```python
from build123d import *

# Parameters (mm, degrees)
F0_R           = 6.1
F1_DEPTH       = 10
F2_W           = 8.5
F2_H           = 45.4
F2_W_2         = 10
F3_DEPTH       = 10
F5_D           = 3.3
F5_CBORE_D     = 6.5
F5_CBORE_DEPTH = 3
F7_DEPTH       = 8.5
F7_DEPTH_BACK  = 18.5
F9_DEPTH       = 45.401


with BuildPart() as f1:
    # F0 (on Right) → F1 (new body)
    with BuildSketch(Plane.YZ):
        with BuildLine():
            Line((22.7, 0), (0, 0))
            Line((0, 0), (-22.7, 0))
            Line((-22.7, 0), (-10, -45))
            ThreePointArc((-10, -45), (0, -35), (10, -45))
            Line((10, -45), (22.7, 0))
        make_face()
        with Locations((0, -10)):
            Circle(F0_R, mode=Mode.SUBTRACT)
        with BuildLine():
            ThreePointArc((10, -45), (0, -35), (-10, -45))
            ThreePointArc((-10, -45), (0, -55), (10, -45))
        make_face()
        with Locations((0, -45)):
            Circle(F0_R, mode=Mode.SUBTRACT)
    extrude(amount=F1_DEPTH)

    # F2 (on face) → F3 (join)
    with BuildSketch(Plane.XY):
        with Locations((14.25, 0)):
            Rectangle(F2_W, F2_H)
        with Locations((5, 0)):
            Rectangle(F2_W_2, F2_H)
        with Locations((-4.25, 0)):
            Rectangle(F2_W, F2_H)
    extrude(amount=F3_DEPTH)

    # F5 (through all)
    with Locations(Plane(origin=(0, 0, 0), x_dir=(1, 0, 0), z_dir=(0, 0, -1))):
        with Locations((-5, 10), (15, 10), (15, -10), (-5, -10)):
            CounterBoreHole(F5_D / 2, F5_CBORE_D / 2, F5_CBORE_DEPTH)

    # F6 (on face) → F7 (join, two sides)
    with BuildSketch(Plane.YZ.offset(10)) as f7_sk:
        with BuildLine():
            Line((21.1, 0), (8.4, -45))
            ThreePointArc((8.4, -45), (0, -53.4), (-8.4, -45))
            Line((-8.4, -45), (-21.1, 0))
            Line((-21.1, 0), (-22.7, 0))
            Line((-22.7, 0), (-10, -45))
            ThreePointArc((-10, -45), (0, -55), (10, -45))
            Line((10, -45), (22.7, 0))
            Line((22.7, 0), (21.1, 0))
        make_face()
    extrude(amount=F7_DEPTH)
    extrude(f7_sk.sketch, amount=-F7_DEPTH_BACK)

    # F8 (on face) → F9 (cut, through all)
    with BuildSketch(Plane.XZ.offset(22.7)):
        Polygon((0, -45), (-8.5, 0), (-8.5, -58.9339546859), (18.5, -58.9339546859), (18.5, 0), (10, -45), (10, -55), (0, -55), align=None)
    extrude(amount=-F9_DEPTH, mode=Mode.SUBTRACT)


solid = f1.part
```
The listing builds one solid part. Answer for the finished solid, in the listing's coordinates (mm). A direction names the side the tool comes from. Round coordinates to 2 decimals unless told otherwise and drop trailing zeros. Write each loop counter-clockwise with the first axis right and the second up, starting at its lowest first coordinate (ties: lowest second). Pieces come first, ordered by that corner, then holes. Notation, with made-up numbers: (-29.5, 9) -> (-12.5, 9) arc R16 ccw to (-12.5, 14) -> close; hole circle Ø6 at (-22, 34.25). An arc over 180 degrees is marked (long way). Answer as a JSON object with one key per item and string values. Group by question number.
Q1. Straight lines are drawn through the part: line 1 along Y through (x, z) = (-5, 2.1); line 2 along X through (y, z) = (10, 1); line 3 along X through (y, z) = (-10, 6.75). For each, find the intervals that lie inside material, in ascending order.
Q2. Section D-D (x = 15) is taken. Write down the section's boundary in (y, z).
Q3. Each of these flat-tipped pins is pushed along its axis until it touches: pin 1 Ø4 at (y, z) = (8, -28) entering from -X; pin 2 Ø2 at (x, y) = (15, 10) entering from +Z; pin 3 Ø2.5 at (x, y) = (-4.5, 7) entering from -Z; pin 4 Ø4 at (x, y) = (-5, -10) entering from -Z. Where does it stop, or does it pass through?
Q4. Section B-B (x = 8.25) is taken. Write down the section's boundary in (y, z).
Q5. Section C-C (z = -10) is taken. Write down the section's boundary in (x, y).
Q6. Which of the six approach directions +Z, -Z, +X, -X, +Y, -Y give full straight-line access (tool end or side, diameter ignored) to faces 1 (the face through (-3.25, 16.25, -17.18)), 2 (the face through (13.476, 10.632, 6.549)), 3 (the face through (16.4, 11.4, 3)), 4 (the face through (13.25, 16.25, -17.19))?
Q7. Section A-A (y = 0) is taken. Write down the section's boundary in (x, z), plus the area to 3 significant figures.
Q8. Determine the mould class of faces 5 (the face through (-8.5, 0, 5)), 6 (the face through (12.3, -17.48, -12.82)), 7 (the face through (4.811, 17.672, -17.815)) for opening direction Y: pulls with the +Y half, pulls with the -Y half, needs draft (parallel to the pull), parting line crosses it, or undercut.
Check values:
{
 "1": {"line 1": "-22.7 to -13.25, -6.75 to 6.75, 13.25 to 22.7", "line 2": "-8.5 to -8.25, -1.75 to 11.75, 18.25 to 18.5", "line 3": "-8.5 to -6.65, -3.35 to 13.35, 16.65 to 18.5"},
 "2": {"outline": "(-22.7, 0) -> (-17.47, -18.53) -> (-15.87, -18.53) -> (-21.1, 0) -> (-13.25, 0) -> (-13.25, 3) -> (-11.65, 3) -> (-11.65, 10) -> (-22.7, 10) -> close; (-8.35, 3) -> (-6.75, 3) -> (-6.75, 0) -> (6.75, 0) -> (6.75, 3) -> (8.35, 3) -> (8.35, 10) -> (-8.35, 10) -> close; (11.65, 3) -> (13.25, 3) -> (13.25, 0) -> (21.1, 0) -> (15.87, -18.53) -> (17.47, -18.53) -> (22.7, 0) -> (22.7, 10) -> (11.65, 10) -> close"},
 "3": {"pin 1": "x = 0", "pin 2": "through", "pin 3": "z = 0", "pin 4": "z = 3"},
 "4": {"outline": "(-22.7, 0) -> (-10, -45) arc R10 ccw to (10, -45) -> (22.7, 0) -> (22.7, 10) -> (-22.7, 10) -> close; hole circle Ø12.2 at (0, -45); hole circle Ø12.2 at (0, -10)"},
 "5": {"outline": "(-6.61, -19.88) -> (16.61, -19.88) -> (16.61, -18.28) -> (10, -18.28) -> (10, -6.1) -> (0, -6.1) -> (0, -18.28) -> (-6.61, -18.28) -> close; (-6.61, 18.28) -> (0, 18.28) -> (0, 6.1) -> (10, 6.1) -> (10, 18.28) -> (16.61, 18.28) -> (16.61, 19.88) -> (-6.61, 19.88) -> close"},
 "6": {"face 1": "-X", "face 2": "+Z, -Z", "face 3": "-Z", "face 4": "+X"},
 "7": {"outline": "(-8.5, 0) -> (0, 0) -> (0, -3.9) -> (10, -3.9) -> (10, 0) -> (18.5, 0) -> (18.5, 10) -> (-8.5, 10) -> close; (0, -55) -> (10, -55) -> (10, -51.1) -> (0, -51.1) -> close; (0, -38.9) -> (10, -38.9) -> (10, -16.1) -> (0, -16.1) -> close", "area": "576 mm^2"},
 "8": {"face 5": "needs draft", "face 6": "undercut", "face 7": "pulls with the +Y half"}
}
